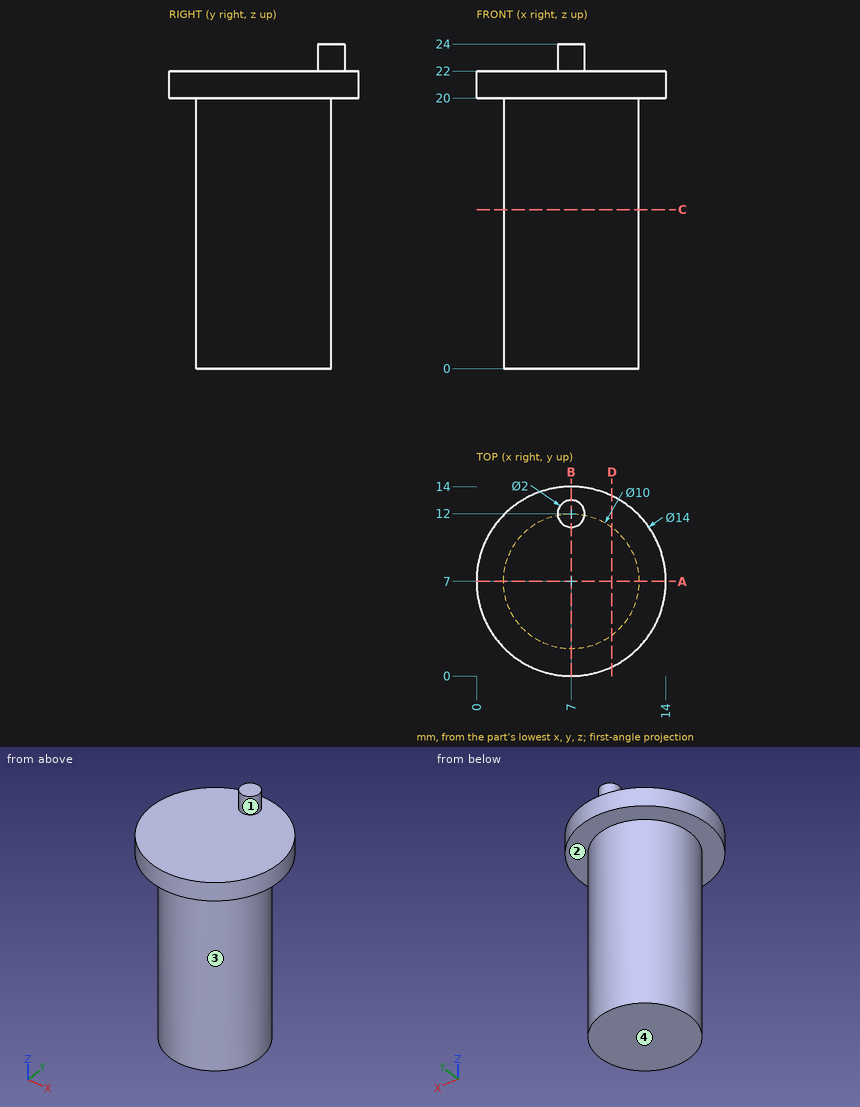
The figure shows three views and two pictorial views of one solid part (mm, origin at its lowest corner). Answer the questions. A direction names the side the tool comes from. Give positions to 0.01 mm unless a question says otherwise; leave off trailing zeros. Write each loop counter-clockwise with the first axis right and the second up, starting at its lowest first coordinate (ties: lowest second). Pieces come first, ordered by that corner, then holes. Notation, with made-up numbers: (22, -31) - (68, -31) arc R10 cw to (68, -23) - close; hole circle Ø7 at (-9.5, -29). An arc over 180 degrees is marked (long way). Use one line per item in the form item = value.
1. A cutting plane is placed at A-A (y = 7). Write down the section's boundary in (x, z).
Filled in:
outline = (0, 20) - (2, 20) - (2, 0) - (12, 0) - (12, 20) - (14, 20) - (14, 22) - (0, 22) - close
2. Consider L1, parallel to Z at x = 12.75, y = 10.75; L2, parallel to Z at x = 6.75, y = 7.25; L3, parallel to X at y = 7.25, z = 10.5. Determine where each line is inside the solid, lowest interval first.
Filled in:
L1 = 20 to 22
L2 = 0 to 22
L3 = 2.01 to 11.99
3. A cutting plane is placed at D-D (x = 10). Write down the section's boundary in (y, z), and give its area (3 significant figures).
Filled in:
outline = (0.68, 20) - (3, 20) - (3, 0) - (11, 0) - (11, 20) - (13.32, 20) - (13.32, 22) - (0.68, 22) - close
area = 185 mm^2
4. Each of these flat-tipped pins is pushed along its axis until it touches: pin 1 Ø8 at (x, z) = (11, 8) entering from -Y; pin 2 Ø4 at (x, z) = (5.5, 18.5) entering from +Y; pin 3 Ø6 at (x, y) = (2.5, 3.5) entering from +Z. Where does it stop, or does it pass through?
Filled in:
pin_1 = 2
pin_2 = 14
pin_3 = 22
5. A cutting plane is placed at B-B (x = 7). Write down the section's boundary in (y, z).
Filled in:
outline = (0, 20) - (2, 20) - (2, 0) - (12, 0) - (12, 20) - (14, 20) - (14, 22) - (13, 22) - (13, 24) - (11, 24) - (11, 22) - (0, 22) - close
6. For the marked faces 3 and 4, determine the directions among +Z, -Z, +X, -X, +Y, -Y from which every point of the face is accessible in a straight line to the end or side of a thin tool.
Filled in:
face_3 = -Z
face_4 = -Z, +X, -X, +Y, -Y
7. A cutting plane is placed at C-C (z = 11.75). Write down the section's boundary in (x, y), and give its area (3 significant figures).
Filled in:
outline = circle Ø10 at (7, 7)
area = 78.5 mm^2
8. Determine the mould class of the marked faces 1 and 2 for opening direction X: released by +X, released by -X, zero draft, split by the parting line, or undercut.
Filled in:
face_1 = split by the parting line
face_2 = zero draft
